Autodesk Inventor part; units mm, degrees
ref_plane "YZ Plane" through (0, 0, 0) normal (1, 0, 0) x (0, 1, 0)
ref_plane "XZ Plane" through (0, 0, 0) normal (0, 1, 0) x (-1, 0, 0)
ref_plane "XY Plane" through (0, 0, 0) normal (0, 0, 1) x (1, 0, 0)
sketch "Sketch1" plane through (0, 0, 0) normal (0, 0, 1) x (1, 0, 0)
  line L0 (-15, 30) -> (15, 30)
  line L1 (15, 30) -> (15, -30)
  line L2 (15, -30) -> (-15, -30)
  line L3 (-15, -30) -> (-15, 30)
  point P0 (0, 0)
  dimension "d0" = 30
  dimension "d1" = 15
  dimension "d2" = 60
  dimension "d3" = 30
extrude "thickness" add sketch "Sketch1" along normal blind 5
sketch "Sketch2" plane through (0, 0, 5) normal (0, 0, 1) x (1, 0, 0)
  line L0 (-15, -30) -> (15, -30)
  point P0 (0, 0)
  point P1 (0, 15)
  dimension "d6" = 45
hole "Hole1" at (0, 15, 5) direction (0, 0, -1) diameter 5 end through all
equation "\"d0\" = sm_varx_squareBarDimension"
equation "\"d4\" = thickness"
equation "\"d7\" = sm_varx_pinPlate_holeDiameter"
equation "\"sm_varx_squareBarDimension\" = 30"
equation "\"thickness\" = sm_varx_pinPlate_thickness"
equation "\"hoop_angle_z\" = 45deg"
equation "\"hoop_bearing_length\" = 5deg"
equation "\"hoop_cable_diam\" = 5"
equation "\"hoop_cable_pulley_diam\" = 22"
equation "\"rack_tooth_addendum\" = 5"
equation "\"rack_tooth_dedendum\" = 5"
equation "\"rack_tooth_thickness\" = 5"
equation "\"secure_arm_angle\" = 20deg"
equation "\"secure_arm_hold_length\" = 35"
equation "\"secure_arm_radii\" = 9"
equation "\"support_baseClamp_platformLengthBuffer\" = 35"
equation "\"support_baseClamp_platformThickness\" = 15"
equation "\"support_baseClamp_platformWidthBuffer\" = 0"
equation "\"support_baseClamp_sleeveHoleDiameter\" = 12"
equation "\"support_baseClamp_sleeveSweepTerminationAngle\" = 55deg"
equation "\"support_baseClamp_thickness\" = 8"
equation "\"support_frame_endHoleBuffer\" = 25"
equation "\"support_frame_squareBarFillet\" = 2"
equation "\"support_frame_squareBarThickness\" = 5"
equation "\"hoop_tabs_thickness\" = 6"
equation "\"hoop_tabs_hole\" = 4"
equation "\"wheelchair_deployed_width\" = 635"
equation "\"wheelchair_deployed_length\" = 1067"
equation "\"wheelchair_deployed_height\" = 914"
equation "\"sm_varx_squareBarThickness\" = 2.5"
equation "\"sm_varx_pinPlate_thickness\" = 5"
equation "\"sm_varx_pinPlate_holeDiameter\" = 5"
properties part number "pinPlate" material "Steel, Galvanized"
Build history of the part. All positions in model axes, mm. Round coordinates to 2 decimals unless told otherwise and drop trailing zeros. Order: outer loops, then holes, each group sorted by start corner. A loop starts at its lowest first (then second) coordinate and runs counter-clockwise, first axis right, second up. Notation, with made-up numbers: M -10,-5 L 43,-5 A26 cw 43,25 Z; hole C 63.25,-29 d4. An arc over 180 degrees is marked long. Use CSV: the item, a comma, the result in double quotes. Start each with the question number.
(1) Drill centre lines: probe 1 along Y at (x, z) = (0, 2); probe 2 along X at (y, z) = (15, 2.4); probe 3 along Y at (x, z) = (-1.5, 0.75). Where is each one in solid material? Low to high.
(2) Cut at B-B on y = 15. List the corners of the cut face in (x, z), then the cut area to 3 significant figures.
(3) Flat gauge pin, fed straight in: P1, Ø4.5, axis at x = 0, y = 15, coming from the -Z side. Where does the tip first touch, or does it go through?
(4) Mould opens along X. For faces 1 (the face through (-0.1, 17.5, 2.5)), 2 (the face through (0, -30, 2)), 3 (the face through (15, 0, 2)) say: +X half, -X half, draft (parallel to the pull), parting line (faces both ways), or undercut.
(5) Cut at A-A on x = 0. List the corners of the cut face in (y, z), then the cut area to 3 significant figures.
Findings:
1,probe 1,"y = -30 to 12.5, 17.5 to 30"
1,probe 2,"x = -15 to -2.5, 2.5 to 15"
1,probe 3,"y = -30 to 13, 17 to 30"
2,outline,"M -15,0 L -2.5,0 L -2.5,5 L -15,5 Z; M 2.5,0 L 15,0 L 15,5 L 2.5,5 Z"
2,area,"125 mm^2"
3,P1,"passes through"
4,face 1,"undercut"
4,face 2,"draft"
4,face 3,"+X half"
5,outline,"M -30,0 L 12.5,0 L 12.5,5 L -30,5 Z; M 17.5,0 L 30,0 L 30,5 L 17.5,5 Z"
5,area,"275 mm^2"
